Input: part model. Units: mm. Frame: model coordinates. Face numbers are marked on the shaded views. A direction names the side the tool comes from. Round coordinates to 2 decimals unless told otherwise and drop trailing zeros. Write each loop counter-clockwise with the first axis right and the second up, starting at its lowest first coordinate (ties: lowest second). Pieces come first, ordered by that corner, then holes. Notation, with made-up numbers: (80, 2) - (112, 2) arc R15 cw to (112, 14) - close; hole circle Ø4 at (-39.5, 28). An arc over 180 degrees is marked (long way). One line per item, written item: value. Start each with the question number.
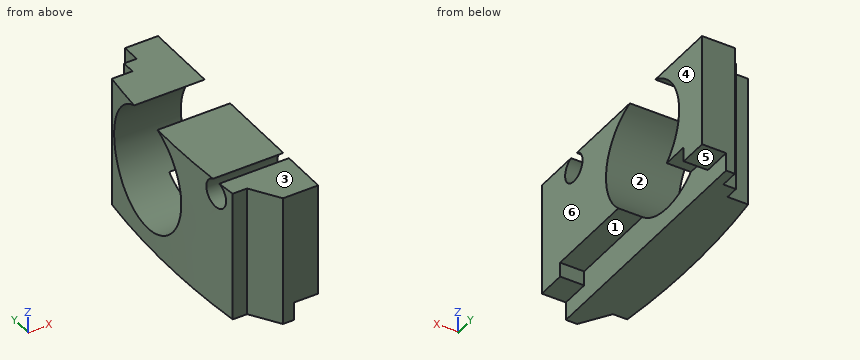
```python
from build123d import *

# Parameters (mm, degrees)
Y_KSEKLIK_EKSTR_ZYON1_DEPTH = 18
IZIM2_W                     = 4.932789915
IZIM2_H                     = 2.5
KES_EKSTR_ZYON1_DEPTH       = 50
IZIM3_R                     = 1.9
KES_EKSTR_ZYON2_DEPTH       = 50
IZIM5_W                     = 2
IZIM5_H                     = 27.034765158
KES_EKSTR_ZYON6_DEPTH       = 3.301675079
IZIM4_R                     = 8
KES_EKSTR_ZYON5_DEPTH       = 50


with BuildPart() as part:
    # Çizim1 → Yükseklik-Ekstrüzyon1 (new body)
    with BuildSketch(Plane.XY):
        with BuildLine():
            Line((-29.072656292, 30.398231235), (-27.345449894, 30.398231235))
            Line((-27.345449894, 30.398231235), (-27.345449894, 32.915968723))
            Line((-27.345449894, 32.915968723), (-22.842394814, 32.915968723))
            Line((-22.842394814, 32.915968723), (-22.842394814, -2.118796435))
            Line((-22.842394814, -2.118796435), (-27.674756319, -2.118796435))
            Line((-27.674756319, -2.118796435), (-30.167426941, 1.750867772))
            Line((-30.167426941, 1.750867772), (-32.139817972, 1.750867772))
            add(Edge.make_bspline(
                [(-32.139817972, 1.750867772), (-32.495187753, 4.885906141), (-32.864718894, 10.152165336), (-32.849440261, 19.124114906), (-32.38234085, 24.914837942), (-31.903618641, 28.562636684)],
                knots=[0.015716623, 0.015716623, 0.015716623, 0.015716623, 0.357537263, 0.585417689, 0.984003614, 0.984003614, 0.984003614, 0.984003614], degree=3))
            Line((-31.903618641, 28.562636684), (-29.072656292, 28.562636684))
            Line((-29.072656292, 28.562636684), (-29.072656292, 30.398231235))
        make_face()
    extrude(amount=Y_KSEKLIK_EKSTR_ZYON1_DEPTH)

    # Çizim2 → Kes-Ekstrüzyon1 (cut)
    with BuildSketch(Plane(origin=(0, -2.118796435, 0), x_dir=(-1, 0, 0), z_dir=(0, -1, 0))):
        with Locations((23.677674935, -1.25)):
            Rectangle(IZIM2_W, IZIM2_H)
    extrude(amount=-KES_EKSTR_ZYON1_DEPTH, mode=Mode.SUBTRACT)

    # Çizim3 → Kes-Ekstrüzyon2 (cut)
    with BuildSketch(Plane(origin=(-22.842394814, 0, 0), x_dir=(0, 0, -1), z_dir=(1, 0, 0))):
        with Locations((-16.2, 4.881203565)):
            Circle(IZIM3_R)
    extrude(amount=-KES_EKSTR_ZYON2_DEPTH, mode=Mode.SUBTRACT)

    # Çizim5 → Kes-Ekstrüzyon6 (cut)
    with BuildSketch(Plane(origin=(-22.842394814, 0, 0), x_dir=(0, 0, -1), z_dir=(1, 0, 0))):
        with Locations((-3.5, 15.398586144)):
            Rectangle(IZIM5_W, IZIM5_H)
    extrude(amount=-KES_EKSTR_ZYON6_DEPTH, mode=Mode.SUBTRACT)

    # Çizim4 → Kes-Ekstrüzyon5 (cut)
    with BuildSketch(Plane(origin=(-22.842394814, 0, 0), x_dir=(0, 0, -1), z_dir=(1, 0, 0))):
        with Locations((-10.5, 19.915968723)):
            Circle(IZIM4_R)
    extrude(amount=-KES_EKSTR_ZYON5_DEPTH, mode=Mode.SUBTRACT)


solid = part.part
```
Q1. Material intervals for probe 1 along Y at (x, z) = (-25.25, 10.5); probe 2 along Y at (x, z) = (-28.25, 15); probe 3 along Y at (x, z) = (-29.5, 16.2), sorted ascending. Write a range as from..to.
Q2. Contact query for flat-ended pins moving along their axis: pin 1 Ø3 at (y, z) = (31.5, 7) entering from -X; pin 2 Ø1 at (x, y) = (-24.5, 10) entering from -Z; pin 3 Ø2 at (x, y) = (-26.5, 10) entering from -Z; pin 4 Ø3.5 at (y, z) = (4.88, 16.2) entering from -X. Output: stop coordinate, or through.
Q3. Access query for the marked faces 5 and 6. Directions: +Z, -Z, +X, -X, +Y, -Y. A direction counts if a zero-diameter tool reaches every point of the face in a straight line with its end or side. Return the directions, or none.
Q4. Cut plane A-A, the plane x = -24.25. Output: boundary loops of the cut face in (y, z).
Q5. Cut plane D-D, the plane y = 1. Output: boundary loops of the cut face in (x, z), and give its area (3 significant figures).
Q6. Cut plane B-B, the plane z = 16. Count the separate pieces of the cut face and the enclosed holes in it, and give its area (3 significant figures).
Q7. Pull-direction query (Z, two-part tool) for the marked faces 1, 2, 3 and 4; classes: pulls with the +Z half, pulls with the -Z half, needs draft (parallel to the pull), parting line crosses it, or undercut.
Q8. Cut plane C-C, the plane x = -28. Output: boundary loops of the cut face in (y, z), and give its area (3 significant figures).
A:
1. probe 1: y = -2.12..11.92, 27.92..32.92
1. probe 2: y = -1.23..3.41, 6.35..13.3, 26.53..30.4
1. probe 3: y = 0.71..2.98, 6.78..14.3, 25.53..28.56
2. pin 1: stops at x = -29.07
2. pin 2: stops at z = 4.5
2. pin 3: stops at z = 0
2. pin 4: passes through
3. face 5: -Z, +X, +Y, -Y
3. face 6: +Z, -Z, +X, +Y, -Y
4. outline: (-2.12, 2.5) - (1.88, 2.5) - (1.88, 4.5) - (14.62, 4.5) arc R8 cw to (17.13, 18) - (5.49, 18) arc R1.9 cw (long way) to (4.27, 18) - (-2.12, 18) - close; (22.7, 18) arc R8 cw to (25.21, 4.5) - (28.92, 4.5) - (28.92, 2.5) - (32.92, 2.5) - (32.92, 18) - close
5. outline: (-29.68, 0) - (-26.14, 0) - (-26.14, 2.5) - (-22.84, 2.5) - (-22.84, 18) - (-29.68, 18) - close
5. area: 115 mm²
6. separate pieces: 3
6. enclosed holes: 0
6. area: 157 mm²
7. face 1: pulls with the -Z half
7. face 2: undercut
7. face 3: pulls with the +Z half
7. face 4: needs draft
8. outline: (-1.61, 0) - (30.4, 0) - (30.4, 18) - (22.7, 18) arc R8 cw (long way) to (17.13, 18) - (5.49, 18) arc R1.9 cw (long way) to (4.27, 18) - (-1.61, 18) - close
8. area: 366 mm²
